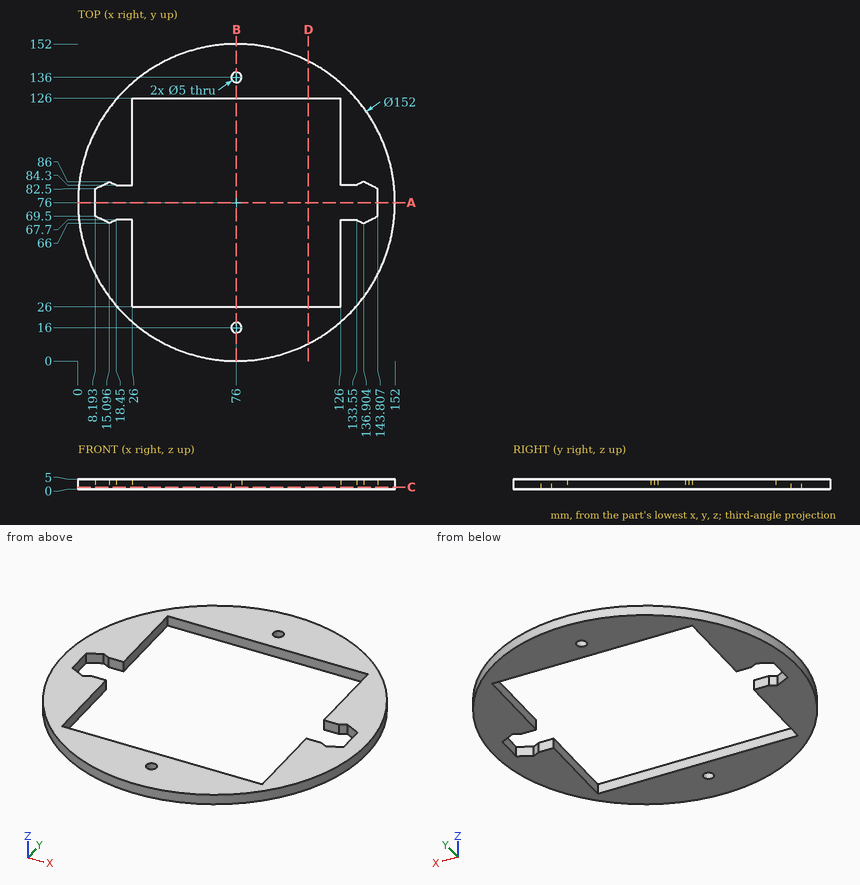
The figure shows three views and two pictorial views of one solid part (mm, origin at its lowest corner). Answer the questions. Coordinates: 2 decimals unless noted, no trailing zeros. Write each loop counter-clockwise with the first axis right and the second up, starting at its lowest first coordinate (ties: lowest second). Pieces come first, ordered by that corner, then holes.
1. The part is cut by section D-D, the plane x = 110.5. Write down the section's boundary in (y, z).
Results list:
outline: (8.28, 0) - (26, 0) - (26, 5) - (8.28, 5) - close; (126, 0) - (143.72, 0) - (143.72, 5) - (126, 5) - close
2. Consider line 1 along Y through (x, z) = (76, 2.8); line 2 along X through (y, z) = (67, 2.15) (1 decimal); line 3 along Y through (x, z) = (75.5, 4.4). Determine where each line is inside the solid, lowest interval first.
Results list:
line 1: y = 0 to 13.5, 18.5 to 26, 126 to 133.5, 138.5 to 152
line 2: x = 0.5 to 13.1, 17.1 to 26, 126 to 134.9, 138.9 to 151.5
line 3: y = 0 to 13.55, 18.45 to 26, 126 to 133.55, 138.45 to 152
3. The part is cut by section C-C, the plane z = 1.1. Write down the section's boundary in (x, y).
Results list:
outline: circle Ø152 at (76, 76); hole (8.19, 69.5) - (15.1, 66) - (18.45, 67.7) - (26, 67.7) - (26, 26) - (126, 26) - (126, 67.7) - (133.55, 67.7) - (136.9, 66) - (143.81, 69.5) - (143.81, 82.5) - (136.9, 86) - (133.55, 84.3) - (126, 84.3) - (126, 126) - (26, 126) - (26, 84.3) - (18.45, 84.3) - (15.1, 86) - (8.19, 82.5) - close; hole circle Ø5 at (76, 16); hole circle Ø5 at (76, 136)
4. Flat-ended cylindrical pins translate along their axes: pin 1 (2.5 mm diameter, centred on x = 61.5, z = 3.5, fed in from -Y); pin 2 (1 mm diameter, centred on x = 82, z = 3.5, fed in from -Y); pin 3 (1.5 mm diameter, centred on y = 73.5, z = 1.5, fed in from +X). Find the tip coordinate at first contact, or state that the pin passes through.
Results list:
pin 1: stops at y = 1.16
pin 2: stops at y = 0.2
pin 3: stops at x = 151.98
5. The part is cut by section A-A, the plane y = 76. Write down the section's boundary in (x, z).
Results list:
outline: (0, 0) - (8.19, 0) - (8.19, 5) - (0, 5) - close; (143.81, 0) - (152, 0) - (152, 5) - (143.81, 5) - close
6. The part is cut by section B-B, the plane x = 76. Write down the section's boundary in (y, z), and give its area (3 significant figures).
Results list:
outline: (0, 0) - (13.5, 0) - (13.5, 5) - (0, 5) - close; (18.5, 0) - (26, 0) - (26, 5) - (18.5, 5) - close; (126, 0) - (133.5, 0) - (133.5, 5) - (126, 5) - close; (138.5, 0) - (152, 0) - (152, 5) - (138.5, 5) - close
area: 210 mm2
